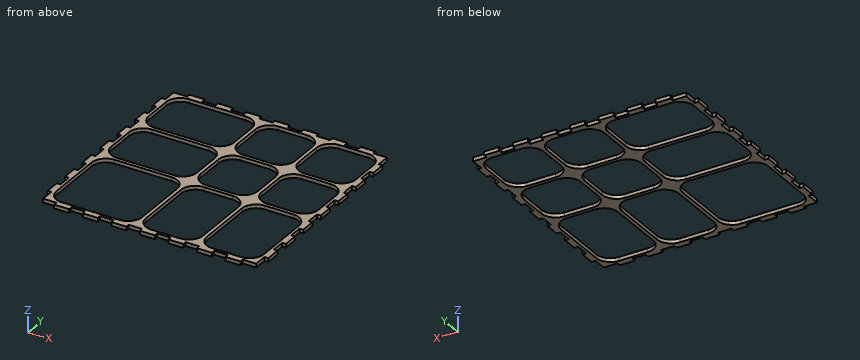
from build123d import *

# Parameters (mm, degrees)
BOSS_EXTRUDE1_DEPTH = 2.5


with BuildPart() as part:
    # Sketch1 → Boss-Extrude1 (new body)
    with BuildSketch(Plane.XY):
        Polygon((-73.5, 0), (-73.5, 5), (-71, 5), (-71, 14), (-73.5, 14), (-73.5, 24), (-71, 24), (-71, 33), (-73.5, 33), (-73.5, 43), (-71, 43), (-71, 52), (-73.5, 52), (-73.5, 62), (-71, 62), (-71, 71), (-62, 71), (-62, 73.5), (-52, 73.5), (-52, 71), (-43, 71), (-43, 73.5), (-33, 73.5), (-33, 71), (-24, 71), (-24, 73.5), (-14, 73.5), (-14, 71), (-5, 71), (-5, 73.5), (5, 73.5), (5, 71), (14, 71), (14, 73.5), (24, 73.5), (24, 71), (33, 71), (33, 73.5), (43, 73.5), (43, 71), (52, 71), (52, 73.5), (62, 73.5), (62, 71), (71, 71), (71, 62), (73.5, 62), (73.5, 52), (71, 52), (71, 43), (73.5, 43), (73.5, 33), (71, 33), (71, 24), (73.5, 24), (73.5, 14), (71, 14), (71, 5), (73.5, 5), (73.5, 0), (73.5, -5), (71, -5), (71, -14), (73.5, -14), (73.5, -24), (71, -24), (71, -33), (73.5, -33), (73.5, -43), (71, -43), (71, -52), (73.5, -52), (73.5, -62), (71, -62), (71, -71), (62, -71), (62, -73.5), (52, -73.5), (52, -71), (43, -71), (43, -73.5), (33, -73.5), (33, -71), (24, -71), (24, -73.5), (14, -73.5), (14, -71), (5, -71), (5, -73.5), (-5, -73.5), (-5, -71), (-14, -71), (-14, -73.5), (-24, -73.5), (-24, -71), (-33, -71), (-33, -73.5), (-43, -73.5), (-43, -71), (-52, -71), (-52, -73.5), (-62, -73.5), (-62, -71), (-71, -71), (-71, -62), (-73.5, -62), (-73.5, -52), (-71, -52), (-71, -43), (-73.5, -43), (-73.5, -33), (-71, -33), (-71, -24), (-73.5, -24), (-73.5, -14), (-71, -14), (-71, -5), (-73.5, -5), align=None)
        with BuildLine():
            Line((-9.5, 59.5), (-9.5, 40.5))
            ThreePointArc((-9.5, 40.5), (-6.717514421, 33.782485579), (0, 31))
            Line((0, 31), (19, 31))
            ThreePointArc((19, 31), (25.717514421, 33.782485579), (28.5, 40.5))
            Line((28.5, 40.5), (28.5, 59.5))
            ThreePointArc((28.5, 59.5), (25.717514421, 66.217514421), (19, 69))
            Line((19, 69), (0, 69))
            ThreePointArc((0, 69), (-6.717514421, 66.217514421), (-9.5, 59.5))
        make_face(mode=Mode.SUBTRACT)
        with BuildLine():
            Line((40.5, 69), (59.5, 69))
            ThreePointArc((59.5, 69), (66.217514421, 66.217514421), (69, 59.5))
            Line((69, 59.5), (69, 40.5))
            ThreePointArc((69, 40.5), (66.217514421, 33.782485579), (59.5, 31))
            Line((59.5, 31), (40.5, 31))
            ThreePointArc((40.5, 31), (33.782485579, 33.782485579), (31, 40.5))
            Line((31, 40.5), (31, 59.5))
            ThreePointArc((31, 59.5), (33.782485579, 66.217514421), (40.5, 69))
        make_face(mode=Mode.SUBTRACT)
        with BuildLine():
            Line((-9.5, 19), (-9.5, 0))
            ThreePointArc((-9.5, 0), (-6.717514421, -6.717514421), (0, -9.5))
            Line((0, -9.5), (19, -9.5))
            ThreePointArc((19, -9.5), (25.717514421, -6.717514421), (28.5, 0))
            Line((28.5, 0), (28.5, 19))
            ThreePointArc((28.5, 19), (25.717514421, 25.717514421), (19, 28.5))
            Line((19, 28.5), (0, 28.5))
            ThreePointArc((0, 28.5), (-6.717514421, 25.717514421), (-9.5, 19))
        make_face(mode=Mode.SUBTRACT)
        with BuildLine():
            Line((31, 19), (31, 0))
            ThreePointArc((31, 0), (33.782485579, -6.717514421), (40.5, -9.5))
            Line((40.5, -9.5), (59.5, -9.5))
            ThreePointArc((59.5, -9.5), (66.217514421, -6.717514421), (69, 0))
            Line((69, 0), (69, 19))
            ThreePointArc((69, 19), (66.217514421, 25.717514421), (59.5, 28.5))
            Line((59.5, 28.5), (40.5, 28.5))
            ThreePointArc((40.5, 28.5), (33.782485579, 25.717514421), (31, 19))
        make_face(mode=Mode.SUBTRACT)
        with BuildLine():
            Line((-69, 19), (-69, 0))
            ThreePointArc((-69, 0), (-66.217514421, -6.717514421), (-59.5, -9.5))
            Line((-59.5, -9.5), (-21.5, -9.5))
            ThreePointArc((-21.5, -9.5), (-14.782485579, -6.717514421), (-12, 0))
            Line((-12, 0), (-12, 19))
            ThreePointArc((-12, 19), (-14.782485579, 25.717514421), (-21.5, 28.5))
            Line((-21.5, 28.5), (-59.5, 28.5))
            ThreePointArc((-59.5, 28.5), (-66.217514421, 25.717514421), (-69, 19))
        make_face(mode=Mode.SUBTRACT)
        with BuildLine():
            Line((-59.5, 69), (-21.5, 69))
            ThreePointArc((-21.5, 69), (-14.782485579, 66.217514421), (-12, 59.5))
            Line((-12, 59.5), (-12, 40.5))
            ThreePointArc((-12, 40.5), (-14.782485579, 33.782485579), (-21.5, 31))
            Line((-21.5, 31), (-59.5, 31))
            ThreePointArc((-59.5, 31), (-66.217514421, 33.782485579), (-69, 40.5))
            Line((-69, 40.5), (-69, 59.5))
            ThreePointArc((-69, 59.5), (-66.217514421, 66.217514421), (-59.5, 69))
        make_face(mode=Mode.SUBTRACT)
        with BuildLine():
            Line((-9.5, -21.5), (-9.5, -59.5))
            ThreePointArc((-9.5, -59.5), (-6.717514421, -66.217514421), (0, -69))
            Line((0, -69), (19, -69))
            ThreePointArc((19, -69), (25.717514421, -66.217514421), (28.5, -59.5))
            Line((28.5, -59.5), (28.5, -21.5))
            ThreePointArc((28.5, -21.5), (25.717514421, -14.782485579), (19, -12))
            Line((19, -12), (0, -12))
            ThreePointArc((0, -12), (-6.717514421, -14.782485579), (-9.5, -21.5))
        make_face(mode=Mode.SUBTRACT)
        with BuildLine():
            Line((40.5, -12), (59.5, -12))
            ThreePointArc((59.5, -12), (66.217514421, -14.782485579), (69, -21.5))
            Line((69, -21.5), (69, -59.5))
            ThreePointArc((69, -59.5), (66.217514421, -66.217514421), (59.5, -69))
            Line((59.5, -69), (40.5, -69))
            ThreePointArc((40.5, -69), (33.782485579, -66.217514421), (31, -59.5))
            Line((31, -59.5), (31, -21.5))
            ThreePointArc((31, -21.5), (33.782485579, -14.782485579), (40.5, -12))
        make_face(mode=Mode.SUBTRACT)
        with BuildLine():
            Line((-59.5, -12), (-21.5, -12))
            ThreePointArc((-21.5, -12), (-14.782485579, -14.782485579), (-12, -21.5))
            Line((-12, -21.5), (-12, -59.5))
            ThreePointArc((-12, -59.5), (-14.782485579, -66.217514421), (-21.5, -69))
            Line((-21.5, -69), (-59.5, -69))
            ThreePointArc((-59.5, -69), (-66.217514421, -66.217514421), (-69, -59.5))
            Line((-69, -59.5), (-69, -21.5))
            ThreePointArc((-69, -21.5), (-66.217514421, -14.782485579), (-59.5, -12))
        make_face(mode=Mode.SUBTRACT)
    extrude(amount=BOSS_EXTRUDE1_DEPTH)


solid = part.part
Check sheet for the modelled part. Datum: model origin and axes. Units: mm. Round coordinates to 2 decimals unless told otherwise and drop trailing zeros. Order: outer loops, then holes, each group sorted by start corner. A loop starts at its lowest first (then second) coordinate and runs counter-clockwise, first axis right, second up. Notation, with made-up numbers: M 31.5,36.25 L 88.5,36.25 A33 ccw 88.5,66.25 Z; hole C 7.25,-28.75 d8. An arc over 180 degrees is marked long. One line per item, written item: value. Start each with the question number.
1. Section check C-C on z = 0.8. Give the number of separate pieces and of enclosed holes in the cut face, and give its area (3 significant figures).
2. Section check A-A on y = 56. Enter the section's corners in (x, z).
3. Scan lines: line 1 along Y through (x, z) = (-30.5, 1.7); line 2 along Y through (x, z) = (56.5, 2.2). Record each from-to range of solid material in increasing order.
4. Gauge pin test, flat ends, axial feed: P1, Ø1.2, axis at y = 72.5, z = 1, coming from the -X side; P2, Ø0.8, axis at x = -73, z = 1.5, coming from the -Y side; P3, Ø1, axis at x = -50.5, z = 1.5, coming from the +Y side. Record the tip position at first contact, or that the pin passes through.
5. Section check B-B on x = -18. Enter the section's corners in (y, z), and give its area (3 significant figures).
Results found:
1. separate pieces: 1
1. enclosed holes: 9
1. area: 3,870 mm^2
2. outline: M -73.5,0 L -69,0 L -69,2.5 L -73.5,2.5 Z; M -12,0 L -9.5,0 L -9.5,2.5 L -12,2.5 Z; M 28.5,0 L 31,0 L 31,2.5 L 28.5,2.5 Z; M 69,0 L 73.5,0 L 73.5,2.5 L 69,2.5 Z
3. line 1: -71 to -69, -12 to -9.5, 28.5 to 31, 69 to 71
3. line 2: -73.5 to -69, -12 to -9.5, 28.5 to 31, 69 to 73.5
4. P1: x = -62
4. P2: y = -62
4. P3: y = 71
5. outline: M -73.5,0 L -68.33,0 L -68.33,2.5 L -73.5,2.5 Z; M -12.67,0 L -8.83,0 L -8.83,2.5 L -12.67,2.5 Z; M 27.83,0 L 31.67,0 L 31.67,2.5 L 27.83,2.5 Z; M 68.33,0 L 73.5,0 L 73.5,2.5 L 68.33,2.5 Z
5. area: 45.0 mm^2
